Verification items for this drawing (mm, ordinates from the low corner). Round coordinates to 2 decimals unless told otherwise and drop trailing zeros. Loops run counter-clockwise (first coordinate to the right, second up) from the corner with the lowest first, then second, coordinate; pieces in that order, holes last. Notation, with made-up numbers: (22, -4.5) -> (45, -4.5) arc R34 cw to (45, 25.5) -> close; hole circle Ø10 at (-35, 13.5). An arc over 180 degrees is marked (long way). One line per question, with ' | ' between items.
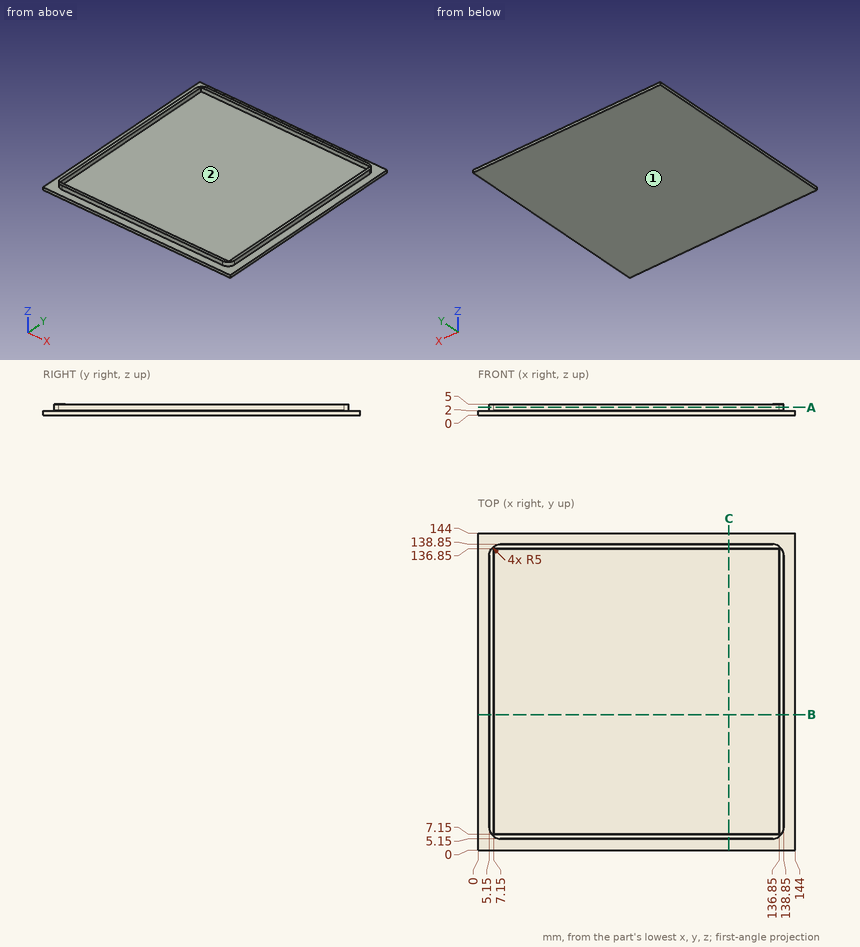
(1) Scan lines: probe 1 along Y at (x, z) = (27, 3.2); probe 2 along Z at (x, y) = (92.5, 88). Record each from-to range of solid material in increasing order.
Answer:
probe 1: y = 5.15 to 7.15, 136.85 to 138.85 | probe 2: z = 0 to 2
(2) Sectioned sample at A-A, the plane z = 3.45. Record the cut outline in (x, y), and give its area (3 significant figures).
Answer:
outline: (5.15, 10.15) arc R5 ccw to (10.15, 5.15) -> (133.85, 5.15) arc R5 ccw to (138.85, 10.15) -> (138.85, 133.85) arc R5 ccw to (133.85, 138.85) -> (10.15, 138.85) arc R5 ccw to (5.15, 133.85) -> close; hole (7.15, 7.15) -> (136.85, 7.15) -> (136.85, 136.85) -> (7.15, 136.85) -> close | area: 1,030 mm2
(3) Mould release check, pull along Y, two halves, no side actions. Record for the marked faces 1 and 2: +Y half, -Y half, draft (parallel to the pull), parting line (faces both ways), or undercut.
Answer:
face 1: draft | face 2: undercut
(4) Go/stop test with flat-tipped pins: pin 1 (1.5 mm diameter, centred on x = 65.5, z = 4, fed in from +Y); pin 2 (1.5 mm diameter, centred on y = 61.5, z = 3, fed in from +X); pin 3 (2.5 mm diameter, centred on y = 75.5, z = 4, fed in from -X). Record where each tip stops, or that it passes through.
Answer:
pin 1: stops at y = 138.85 | pin 2: stops at x = 138.85 | pin 3: stops at x = 5.15
(5) Sectioned sample at B-B, the plane y = 61.5. Record the cut outline in (x, z).
Answer:
outline: (0, 0) -> (144, 0) -> (144, 2) -> (138.85, 2) -> (138.85, 5) -> (136.85, 5) -> (136.85, 2) -> (7.15, 2) -> (7.15, 5) -> (5.15, 5) -> (5.15, 2) -> (0, 2) -> close
